Design review of the part built by this model. Coordinates are the model's own, in mm. Face numbers are marked on the shaded views. A direction names the side the tool comes from. Give positions to 0.01 mm unless a question says otherwise; leave off trailing zeros. Order: outer loops, then holes, each group sorted by start corner. A loop starts at its lowest first (then second) coordinate and runs counter-clockwise, first axis right, second up. Notation, with made-up numbers: (-26.75, 45) -> (2.25, 45) arc R35 ccw to (2.25, 81) -> close; hole circle Ø1 at (8.25, -36). An arc over 180 degrees is marked (long way). One line per item, written item: value. Start each with the question number.
1) Consider section B-B (x = 0). State the section outline as (y, z) points, plus the area to 3 significant figures.
2) For pin 1 (10 mm diameter, centred on x = 2, z = 65.5, fed in from -Y); pin 2 (2 mm diameter, centred on y = 0.5, z = 134, fed in from +X); pin 3 (4 mm diameter, centred on x = 6, y = 16.5, fed in from -Z); pin 4 (5 mm diameter, centred on y = -16.5, z = 74, fed in from +X), all flat-tipped, find the tip position at first contact; note any pin that passes through.
3) Consider section D-D (z = 22). State the section outline as (x, y) points.
4) Tool access review of the marked faces 1 and 2: name each direction out of +Z, -Z, +X, -X, +Y, -Y from which nothing blocks a thin tool from reaching the whole face with its end or side.
5) Consider section A-A (z = 55). State the section outline as (x, y) points.
6) Wall thickness on line 1 along Y through (x, z) = (0, 94); line 2 along X through (y, z) = (0, 129): over which ranges is each line inside the solid? List them lowest first. Write a range as from..to.
from build123d import *


with BuildPart() as f1:
    # F0 (on Front) → F1 (revolve)
    with BuildSketch(Plane.XZ):
        with BuildLine():
            Line((-10, 0), (-5, 0))
            Line((-5, 0), (-5, 87.784544))
            Line((-5, 87.784544), (-5, 95))
            Line((-5, 95), (-5, 190))
            Line((-5, 190), (0, 190))
            Line((0, 190), (0, 220))
            Line((0, 220), (-14.767565, 220))
            ThreePointArc((-14.767565, 220), (-18.382478, 218.454331), (-19.762407, 214.772962))
            Line((-19.762407, 214.772962), (-14.318182, 95))
            Line((-14.318182, 95), (-22.129804, 95))
            Line((-22.129804, 95), (-22.129804, 87.784544))
            Line((-22.129804, 87.784544), (-13.990207, 87.784544))
            Line((-13.990207, 87.784544), (-10, 0))
        make_face()
    revolve(axis=Axis((0, 0, 135.638863), (0, 0, 1)))


solid = f1.part
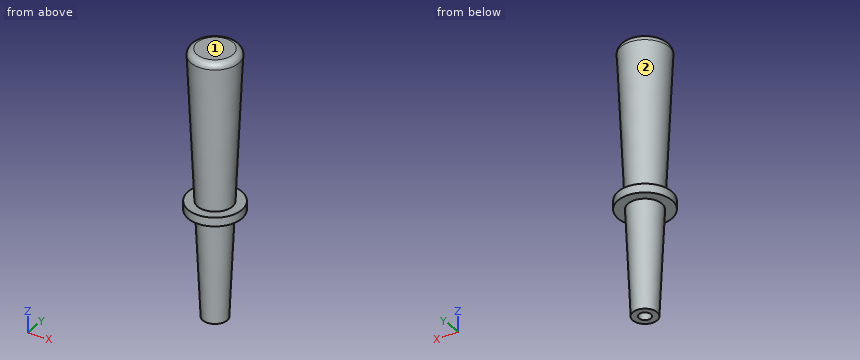
Checked values:
1. outline: (-22.13, 87.78) -> (-13.99, 87.78) -> (-10, 0) -> (-5, 0) -> (-5, 190) -> (5, 190) -> (5, 0) -> (10, 0) -> (13.99, 87.78) -> (22.13, 87.78) -> (22.13, 95) -> (14.32, 95) -> (19.76, 214.77) arc R5 ccw to (14.77, 220) -> (-14.77, 220) arc R5 ccw to (-19.76, 214.77) -> (-14.32, 95) -> (-22.13, 95) -> close
1. area: 4,800 mm^2
2. pin 1: stops at y = -13.19
2. pin 2: stops at x = 16.13
2. pin 3: stops at z = 87.78
2. pin 4: passes through
3. outline: circle Ø22 at (0, 0); hole circle Ø10 at (0, 0)
4. face 1: +Z, +X, -X, +Y, -Y
4. face 2: none
5. outline: circle Ø25 at (0, 0); hole circle Ø10 at (0, 0)
6. line 1: y = -22.13..-5, 5..22.13
6. line 2: x = -15.86..-5, 5..15.86
